Here's how the part is built. I have some questions about the finished solid (model axes, mm). Face numbers are marked on the shaded views. A direction names the side the tool comes from. Give positions to 0.01 mm unless a question says otherwise; leave off trailing zeros. Loops run counter-clockwise (first coordinate to the right, second up) from the corner with the lowest first, then second, coordinate; pieces in that order, holes last. Notation, with made-up numbers: (87, -6.75) -> (102, -6.75) arc R10 cw to (102, 7.25) -> close; hole circle Ø10 at (9, 4). An arc over 180 degrees is marked (long way). Answer in a Markdown table with one row per item. Add a question column.
Item 1: If we section it at A-A (x = 0): Give the number of separate pieces and of enclosed holes in the cut face, then the cut area to 3 significant figures.
Item 2: If we section it at B-B (x = 23): Write out the boundary of the cut face in (y, z).
Item 3: We'd pull the mould along X, two halves only. Please class the marked faces 3 and 4: released by +X, released by -X, zero draft, split by the parting line, or undercut.
Item 4: Which directions (+Z, -Z, +X, -X, +Y, -Y) give clear straight access to the entire face, cutting with the end or side of a thin tool? Please do the marked faces 1 and 2.
Item 5: For P1, Ø9, axis at x = 0, y = 0.26, coming from the -Z side; P2, Ø1, axis at x = 0.5, z = 1.5, coming from the +Y side; P3, Ø1, axis at y = 0.5, z = 2, coming from the +X side, each with a flat end and sliding along its axis, tell me the tip position at first contact or that it passes through.
Item 6: If we section it at D-D (x = 16.5): Write out the boundary of the cut face in (y, z), then the cut area to 3 significant figures.
Item 7: If I drill on line 1 (X direction, y = 8.5, z = 0.7); line 2 (X direction, y = -2, z = 2.1); line 3 (Z direction, x = -20, y = -24.5), over which ranges is the centre line in solid material (lowest first)?
Autodesk Inventor part; units mm, degrees
ref_plane "YZ Plane" through (0, 0, 0) normal (1, 0, 0) x (0, 1, 0)
ref_plane "XZ Plane" through (0, 0, 0) normal (0, 1, 0) x (-1, 0, 0)
ref_plane "XY Plane" through (0, 0, 0) normal (0, 0, 1) x (1, 0, 0)
sketch "Sketch1" plane through (0, 0, 0) normal (0, 0, 1) x (1, 0, 0)
  circle A0 centre (0, 0) radius 31.1101
extrude "Extrusion1" add sketch "Sketch1" along normal blind 2.794
sketch "Sketch2" plane through (0, 0, 0) normal (0, 0, -1) x (-1, 0, 0)
  circle A0 centre (0, 0) radius 31.75
  dimension "d2" = 63.5
extrude "Extrusion2" add sketch "Sketch2" along normal blind 0.254
sketch "Sketch3" plane through (0, 0, 2.794) normal (0, 0, 1) x (1, 0, 0)
  circle A0 centre (0, 0) radius 31.75
  dimension "d5" = 63.5
extrude "Extrusion3" add sketch "Sketch3" along normal blind 0.254
sketch "Sketch4" plane through (0, 0, -0.254) normal (0, 0, -1) x (-1, 0, 0)
  arc A0 (-1.5256, 7.6067) -> (1.5256, 7.6067) centre (0, 8.5367) ccw
  line L0 (-1.5256, 7.6067) -> (-10.0877, 14.0155)
  arc A1 (-10.0877, 14.0155) -> (-14.0155, 10.0877) centre (-11.7691, 11.7691) ccw
  line L1 (-14.0155, 10.0877) -> (-7.6067, 1.5256)
  arc A2 (-7.6067, -1.5256) -> (-7.6067, 1.5256) centre (-8.5367, 0) ccw
  line L2 (-7.6067, -1.5256) -> (-14.0155, -10.0877)
  arc A3 (-14.0155, -10.0877) -> (-10.0877, -14.0155) centre (-11.7691, -11.7691) ccw
  line L3 (-10.0877, -14.0155) -> (-1.5256, -7.6067)
  arc A4 (1.5256, -7.6067) -> (-1.5256, -7.6067) centre (0, -8.5367) ccw
  line L4 (1.5256, -7.6067) -> (10.0877, -14.0155)
  arc A5 (10.0877, -14.0155) -> (14.0155, -10.0877) centre (11.7691, -11.7691) ccw
  line L5 (14.0155, -10.0877) -> (7.6067, -1.5256)
  arc A6 (7.6067, 1.5256) -> (7.6067, -1.5256) centre (8.5367, 0) ccw
  line L6 (7.6067, 1.5256) -> (14.0155, 10.0877)
  arc A7 (14.0155, 10.0877) -> (10.0877, 14.0155) centre (11.7691, 11.7691) ccw
  line L7 (10.0877, 14.0155) -> (1.5256, 7.6067)
  circle A8 centre (0, 0) radius 5.27
  circle A9 centre (-4.9144, 4.9144) radius 0.75
  circle A10 centre (-7.3893, 7.3893) radius 0.75
  circle A11 centre (-9.8641, 9.8641) radius 0.75
  circle A12 centre (-12.339, 12.339) radius 0.75
  circle A13 centre (-4.9144, -4.9144) radius 0.75
  circle A14 centre (-7.3893, -7.3893) radius 0.75
  circle A15 centre (-9.8641, -9.8641) radius 0.75
  circle A16 centre (-12.339, -12.339) radius 0.75
  circle A17 centre (4.9144, -4.9144) radius 0.75
  circle A18 centre (7.3893, -7.3893) radius 0.75
  circle A19 centre (9.8641, -9.8641) radius 0.75
  circle A20 centre (12.339, -12.339) radius 0.75
  circle A21 centre (4.9144, 4.9144) radius 0.75
  circle A22 centre (7.3893, 7.3893) radius 0.75
  circle A23 centre (9.8641, 9.8641) radius 0.75
  circle A24 centre (12.339, 12.339) radius 0.75
extrude "Extrusion4" cut sketch "Sketch4" against normal blind 1.3335 contours A0 L7 A7 L6 A6 L5 A5 L4 A4 L3 A3 L2 A2 L1 A1 L0 | A8 | A9 | A10 | A11 | A12 | A13 | A14 | A15 | A16 | A17 | A18 | A19 | A20 | A21 | A22 | A23 | A24
sketch "Sketch5" plane through (0, 0, -0.254) normal (0, 0, -1) x (-1, 0, 0)
  point P0 (0, 0)
hole "Hole1" at (0, 0, -0.254) direction (0, 0, 1) diameter 10.541 depth 1.5875
hole "Hole2" at (0.0046, 0.2595, 1.3335) direction (0, 0, 1) diameter 10.541 depth 0.254
sketch "Sketch6" plane through (0, 0, -0.254) normal (0, 0, -1) x (-1, 0, 0)
  line L0 (-6.735, 18.6967) -> (7.235, 18.6967)
  line L1 (10.41, 21.8717) -> (10.41, 24.4117)
  line L2 (7.235, 27.5867) -> (-6.735, 27.5867)
  line L3 (-9.91, 24.4117) -> (-9.91, 21.8717)
  line L4 (21.8717, 10.2323) -> (24.4117, 10.2323)
  line L5 (27.5867, 7.0573) -> (27.5867, -6.9127)
  line L6 (24.4117, -10.0877) -> (21.8717, -10.0877)
  line L7 (18.6967, -6.9127) -> (18.6967, 7.0573)
  arc A0 (7.6067, 1.5256) -> (7.6067, -1.5256) centre (8.5367, 0) ccw
  arc A1 (-1.5256, 7.6067) -> (1.5256, 7.6067) centre (0, 8.5367) ccw
  line L8 (-21.8717, -10.0877) -> (-24.4117, -10.0877)
  line L9 (-27.5867, -6.9127) -> (-27.5867, 7.0573)
  line L10 (-24.4117, 10.2323) -> (-21.8717, 10.2323)
  line L11 (-18.6967, 7.0573) -> (-18.6967, -6.9127)
  arc A2 (-7.6067, -1.5256) -> (-7.6067, 1.5256) centre (-8.5367, 0) ccw
  line L12 (7.235, -18.6967) -> (-6.735, -18.6967)
  line L13 (-9.91, -21.8717) -> (-9.91, -24.4117)
  line L14 (-6.735, -27.5867) -> (7.235, -27.5867)
  line L15 (10.41, -24.4117) -> (10.41, -21.8717)
  arc A3 (1.5256, -7.6067) -> (-1.5256, -7.6067) centre (0, -8.5367) ccw
  arc A4 (27.5867, 7.0573) -> (24.4117, 10.2323) centre (24.4117, 7.0573) ccw
  arc A5 (24.4117, -10.0877) -> (27.5867, -6.9127) centre (24.4117, -6.9127) ccw
  arc A6 (18.6967, -6.9127) -> (21.8717, -10.0877) centre (21.8717, -6.9127) ccw
  arc A7 (21.8717, 10.2323) -> (18.6967, 7.0573) centre (21.8717, 7.0573) ccw
  arc A8 (7.235, -27.5867) -> (10.41, -24.4117) centre (7.235, -24.4117) ccw
  arc A9 (-9.91, -24.4117) -> (-6.735, -27.5867) centre (-6.735, -24.4117) ccw
  arc A10 (-6.735, -18.6967) -> (-9.91, -21.8717) centre (-6.735, -21.8717) ccw
  arc A11 (10.41, -21.8717) -> (7.235, -18.6967) centre (7.235, -21.8717) ccw
  arc A12 (-6.735, 27.5867) -> (-9.91, 24.4117) centre (-6.735, 24.4117) ccw
  arc A13 (10.41, 24.4117) -> (7.235, 27.5867) centre (7.235, 24.4117) ccw
  arc A14 (-9.91, 21.8717) -> (-6.735, 18.6967) centre (-6.735, 21.8717) ccw
  arc A15 (7.235, 18.6967) -> (10.41, 21.8717) centre (7.235, 21.8717) ccw
  arc A16 (-27.5867, -6.9127) -> (-24.4117, -10.0877) centre (-24.4117, -6.9127) ccw
  arc A17 (-24.4117, 10.2323) -> (-27.5867, 7.0573) centre (-24.4117, 7.0573) ccw
  arc A18 (-21.8717, -10.0877) -> (-18.6967, -6.9127) centre (-21.8717, -6.9127) ccw
  arc A19 (-18.6967, 7.0573) -> (-21.8717, 10.2323) centre (-21.8717, 7.0573) ccw
  circle A20 centre (0, 0) radius 1.27
  point P0 (-9.91, 18.6967)
  point P1 (10.41, 27.5867)
  point P2 (10.41, 18.6967)
  point P3 (-9.91, 27.5867)
  point P4 (18.6967, 10.2323)
  point P5 (27.5867, -10.0877)
  point P6 (27.5867, 10.2323)
  point P7 (18.6967, -10.0877)
  point P8 (-18.6967, -10.0877)
  point P9 (-27.5867, 10.2323)
  point P10 (-27.5867, -10.0877)
  point P11 (-18.6967, 10.2323)
  point P12 (10.41, -18.6967)
  point P13 (-9.91, -27.5867)
  point P14 (-9.91, -18.6967)
  point P15 (10.41, -27.5867)
  dimension "d26" = 10.16
  dimension "d27" = 8.89
  dimension "d28" = 20.32
  dimension "d29" = 10.16
  dimension "d30" = 20.32
  dimension "d31" = 8.89
  dimension "d32" = 10.16
  dimension "d33" = 20.32
  dimension "d34" = 8.89
  dimension "d35" = 10.16
  dimension "d36" = 8.89
  dimension "d37" = 20.32
  dimension "d40" = 3.175
  dimension "d41" = 2.54
extrude "Extrusion5" cut sketch "Sketch6" against normal blind 38.1 contours A14 L3 A12 L2 A13 L1 A15 L0 | L4 A4 L5 A5 L6 A6 L7 A7 | L8 A16 L9 A17 L10 A19 L11 A18 | A11 L15 A8 L14 A9 L13 A10 L12
sketch "Sketch7" plane through (0.0046, 0.2595, 1.5875) normal (0, 0, -1) x (-1, 0, 0)
  circle A0 centre (0, 0) radius 1.27
  point P0 (0.0046, -0.2595)
  dimension "d42" = 2.54
extrude "Extrusion6" cut sketch "Sketch7" along normal mid plane 25.4
sketch "Sketch8" plane through (0.0046, 0.2595, 1.5875) normal (0, 0, -1) x (-1, 0, 0)
  circle A0 centre (0, 0) radius 5.4861
  point P0 (0.0046, -0.2595)
extrude "Extrusion7" cut sketch "Sketch8" along normal blind 1.5875
sketch "Sketch9" plane through (0.0046, 0.2595, 1.5875) normal (0, 0, -1) x (-1, 0, 0)
  circle A0 centre (0, 0) radius 5.715
  point P0 (0.0046, -0.2595)
  dimension "d47" = 11.43
extrude "Extrusion8" cut sketch "Sketch9" along normal blind 25.4
properties part number "RTS  Wheel"
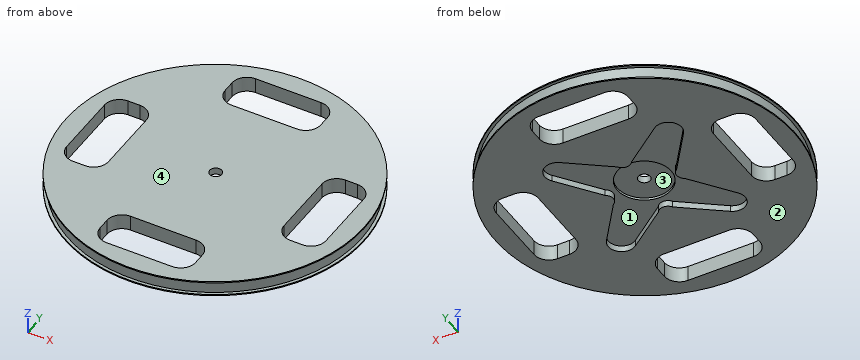
Recorded:
| question | item | result |
|---|---|---|
| 1 | separate pieces | 4 |
| 1 | enclosed holes | 0 |
| 1 | area | 120 mm^2 |
| 2 | outline | (-21.89, -0.25) -> (-10.09, -0.25) -> (-10.09, 3.05) -> (-21.89, 3.05) -> (-21.89, 2.79) -> (-20.95, 2.79) -> (-20.95, 0) -> (-21.89, 0) -> close; (10.23, -0.25) -> (21.89, -0.25) -> (21.89, 0) -> (20.95, 0) -> (20.95, 2.79) -> (21.89, 2.79) -> (21.89, 3.05) -> (10.23, 3.05) -> close |
| 3 | face 3 | undercut |
| 3 | face 4 | zero draft |
| 4 | face 1 | -Z |
| 4 | face 2 | -Z, +X, -X, +Y, -Y |
| 5 | P1 | stops at z = 1.59 |
| 5 | P2 | stops at y = 31.11 |
| 5 | P3 | stops at x = 31.11 |
| 6 | outline | (-27.13, -0.25) -> (27.13, -0.25) -> (27.13, 0) -> (26.37, 0) -> (26.37, 2.79) -> (27.13, 2.79) -> (27.13, 3.05) -> (-27.13, 3.05) -> (-27.13, 2.79) -> (-26.37, 2.79) -> (-26.37, 0) -> (-27.13, 0) -> close |
| 6 | area | 175 mm^2 |
| 7 | line 1 | x = -29.93 to -27.24, -19.04 to -12.83, -2.72 to 2.72, 12.83 to 19.04, 27.24 to 29.93 |
| 7 | line 2 | x = -31.05 to -27.59, -18.7 to 18.7, 27.59 to 31.05 |
| 7 | line 3 | z = -0.25 to 0, 2.79 to 3.05 |
